Build history of the part. All positions in model axes, mm. A direction names the side the tool comes from. Round coordinates to 2 decimals unless told otherwise and drop trailing zeros. Write each loop counter-clockwise with the first axis right and the second up, starting at its lowest first coordinate (ties: lowest second). Pieces come first, ordered by that corner, then holes. Notation, with made-up numbers: M -38.75,-30 L -30.75,-30 A29 cw -30.75,-5 Z; hole C -1,81.25 d11. An arc over 180 degrees is marked long. Write item = value, one per line.
from build123d import *

# Parameters (mm, degrees)
F0_W           = 1311.275
F0_H           = 508
F0_W_2         = 1235.075
F0_H_2         = 431.8
F1_DEPTH       = 19.05
F4_D           = 5.1054
F4_DEPTH       = 16.51
F4_TIP         = 1.5338169022
F4_ON_F3_D     = 5.1054
F4_ON_F3_DEPTH = 16.51
F4_ON_F3_TIP   = 1.5338169022


with BuildPart() as f1:
    # F0 (on Top) → F1 (new body, symmetric)
    with BuildSketch(Plane.XY):
        Rectangle(F0_W, F0_H)
        Rectangle(F0_W_2, F0_H_2, mode=Mode.SUBTRACT)
    extrude(amount=F1_DEPTH, both=True)

    # F4
    with Locations(Plane.YZ.offset(655.6375)):
        with Locations((57.15, 0), (107.95, 0), (-196.85, 0), (-247.65, 0), (-44.45, 0), (-95.25, 0)):
            Hole(F4_D / 2, depth=F4_DEPTH)
            with Locations((0, 0, -(F4_DEPTH + F4_TIP / 2))):  # 118° drill point
                Cone(0, F4_D / 2, F4_TIP, mode=Mode.SUBTRACT)

    # F4 on F3
    with Locations(Plane(origin=(-655.6375, 0, 0), x_dir=(0, -1, 0), z_dir=(-1, 0, 0))):
        with Locations((247.65, 0), (196.85, 0), (-76.2, 0), (-127, 0)):
            Hole(F4_ON_F3_D / 2, depth=F4_ON_F3_DEPTH)
            with Locations((0, 0, -(F4_ON_F3_DEPTH + F4_ON_F3_TIP / 2))):  # 118° drill point
                Cone(0, F4_ON_F3_D / 2, F4_ON_F3_TIP, mode=Mode.SUBTRACT)


solid = f1.part
1. Flat gauge pins, fed straight in: pin 1 (4.5 mm diameter, centred on y = 57.15, z = 0, fed in from +X); pin 2 (3 mm diameter, centred on y = 76.2, z = 0, fed in from -X) (3 decimals); pin 3 (3 mm diameter, centred on y = -247.65, z = 0, fed in from +X) (3 decimals). Where does each tip first touch, or does it go through?
Responses:
pin_1 = 638.95
pin_2 = -638.495
pin_3 = 638.495
2. Band-saw the part on A-A (x = -152). List the corners of the cut face in (y, z).
Responses:
outline = M -254,-19.05 L -215.9,-19.05 L -215.9,19.05 L -254,19.05 Z; M 215.9,-19.05 L 254,-19.05 L 254,19.05 L 215.9,19.05 Z
3. Tool access for faces 1 (the face through (617.538, -3, 0)), 2 (the face through (-9, -254, 0)): list every direction of +Z, -Z, +X, -X, +Y, -Y with a clear straight run to the whole face (end or side of a thin tool).
Responses:
face_1 = +Z, -Z
face_2 = +Z, -Z, +X, -X, -Y
4. Probe probe 1 along Y at (x, z) = (-645.5, 0); probe 2 along Z at (x, y) = (643, 107); probe 3 along X at (y, z) = (213.5, -12). List the from-to ranges inside material, lowest first.
Responses:
probe_1 = -254 to -250.2, -245.1 to -199.4, -194.3 to 73.65, 78.75 to 124.45, 129.55 to 254
probe_2 = -19.05 to -2.37, 2.37 to 19.05
probe_3 = -655.64 to -617.54, 617.54 to 655.64
5. Band-saw the part on B-B (y = 143.5). List the corners of the cut face in (x, z).
Responses:
outline = M -655.64,-19.05 L -617.54,-19.05 L -617.54,19.05 L -655.64,19.05 Z; M 617.54,-19.05 L 655.64,-19.05 L 655.64,19.05 L 617.54,19.05 Z
6. Band-saw the part on C-C (z = 12). List the corners of the cut face in (x, y), plus the area to 3 significant figures.
Responses:
outline = M -655.64,-254 L 655.64,-254 L 655.64,254 L -655.64,254 Z; hole M -617.54,-215.9 L 617.54,-215.9 L 617.54,215.9 L -617.54,215.9 Z
area = 133,000 mm²
7. Mould opens along X. For faces 3 (the face through (-9, 254, 0)), 4 (the face through (-9, -215.9, 0)), 5 (the face through (-655.638, -4, 0)), 6 (the face through (-9, 215.9, 0)) say: pulls with the +X half, pulls with the -X half, needs draft (parallel to the pull), parting line crosses it, or undercut.
Responses:
face_3 = needs draft
face_4 = undercut
face_5 = pulls with the -X half
face_6 = undercut
